The listing builds one solid part. Answer for the finished solid, in the listing's coordinates (mm). Round coordinates to 2 decimals unless told otherwise and drop trailing zeros. Order: outer loops, then holes, each group sorted by start corner. A loop starts at its lowest first (then second) coordinate and runs counter-clockwise, first axis right, second up. Notation, with made-up numbers: (76, 20.5) - (83, 20.5) arc R15 ccw to (83, 49.5) - close; hole circle Ø4 at (-9, 42.25). An arc over 180 degrees is marked (long way). Use CSV: the item, a comma, the result in double quotes. Start each with the question number.
Item 1: Find section A-A, the plane z = 580. Give the vertices of the cut face in (x, y), plus the area to 3 significant figures.
Item 2: Find section D-D, the plane y = 0. Count the separate pieces of the cut face and the enclosed holes in it, plus the area to 3 significant figures.
Item 3: A flat-ended cylindrical pin translates along its axis: P1, Ø6, axis at y = 0, z = 130, coming from the -X side. Find the tip coordinate at first contact, or state that the pin passes through.
Item 4: Find section C-C, the plane z = 329. Give the vertices of the cut face in (x, y).
Item 5: Straight lines are drawn through the part: line 1 along Y through (x, z) = (5, 413); line 2 along Y through (x, z) = (18.6, 490); line 3 along X through (y, z) = (4.75, 265). For each, find the intervals that lie inside material, in ascending order. Write a range as [from, to].
Item 6: Find section B-B, the plane x = -2. Give the vertices of the cut face in (y, z), plus the area to 3 significant figures.
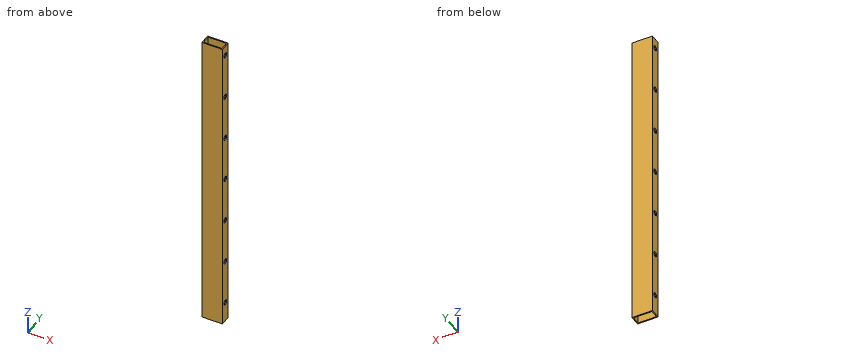
Autodesk Inventor part; units mm, degrees
ref_plane "YZ Plane" through (0, 0, 0) normal (1, 0, 0) x (0, 1, 0)
ref_plane "XZ Plane" through (0, 0, 0) normal (0, 1, 0) x (-1, 0, 0)
ref_plane "XY Plane" through (0, 0, 0) normal (0, 0, 1) x (1, 0, 0)
sketch "Sketch1" plane through (0, 0, 0) normal (0, 0, 1) x (1, 0, 0)
  line L0 (-20, 10) -> (20, 10)
  line L1 (20, 10) -> (20, -10)
  line L2 (20, -10) -> (-20, -10)
  line L3 (-20, -10) -> (-20, 10)
  line L4 (-20, 10) -> (20, -10) construction
  line L5 (18, 8) -> (-18, 8)
  line L6 (-18, 8) -> (-18, -8)
  line L7 (-18, -8) -> (18, -8)
  line L8 (18, -8) -> (18, 8)
  point P0 (0, 0)
  point P1 (0, 0)
  dimension "d0" = 40
  dimension "d1" = 20
  dimension "d4" = 2
extrude "Extrusion1" add sketch "Sketch1" along normal blind 600
sketch "Sketch2" plane through (0, 0, 0) normal (1, 0, 0) x (0, 1, 0)
  line L0 (-10, 0) -> (10, 0)
  line L1 (10, 0) -> (10, 600) construction
  line L2 (-10, 600) -> (10, 600)
  line L3 (-10, 0) -> (-10, 600) construction
  circle A0 centre (0, 580) radius 5
  point P0 (0, 0)
  point P1 (0, 600)
  dimension "d5" = 10
  dimension "d6" = 20
extrude "Extrusion2" cut sketch "Sketch2" along normal through all both and the other way through all
pattern_linear "Rectangular Pattern1" count 7 spacing 90 along (0, 0, -1) of "Extrusion2"
properties part number "Wash way double"
Worked out:
1,outline,"(-20, -10) - (20, -10) - (20, -5) - (18, -5) - (18, -8) - (-18, -8) - (-18, -5) - (-20, -5) - close; (-20, 5) - (-18, 5) - (-18, 8) - (18, 8) - (18, 5) - (20, 5) - (20, 10) - (-20, 10) - close"
1,area,"184 mm²"
2,separate pieces,"16"
2,enclosed holes,"0"
2,area,"2,120 mm²"
3,P1,"passes through"
4,outline,"(-20, -10) - (20, -10) - (20, 10) - (-20, 10) - close; hole (-18, -8) - (18, -8) - (18, 8) - (-18, 8) - close"
5,line 1,"y = [-10, -8], [8, 10]"
5,line 2,"y = [-10, -5], [5, 10]"
5,line 3,"x = [-20, -18], [18, 20]"
6,outline,"(-10, 0) - (-8, 0) - (-8, 600) - (-10, 600) - close; (8, 0) - (10, 0) - (10, 600) - (8, 600) - close"
6,area,"2,400 mm²"
